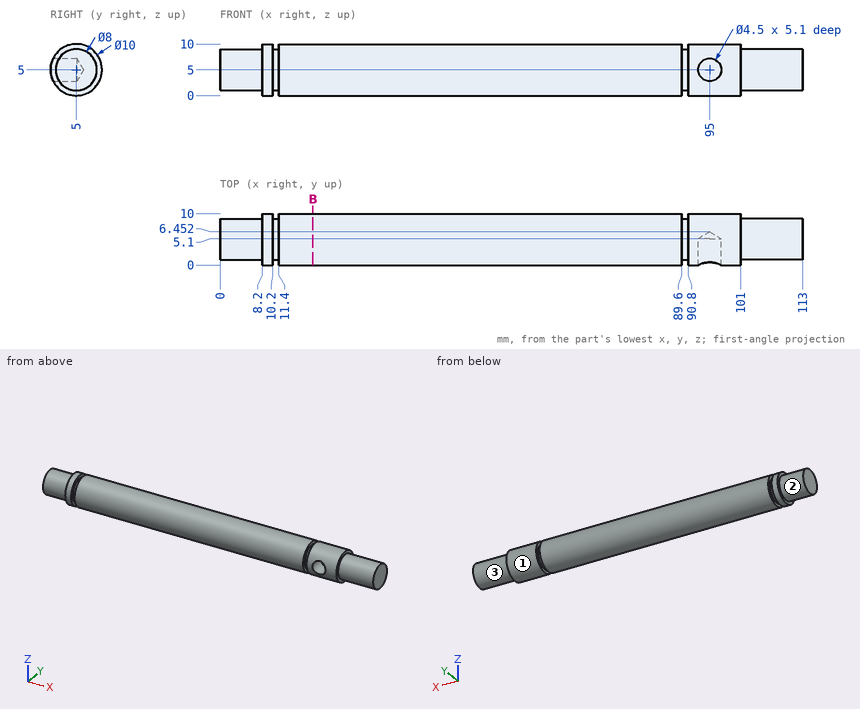
Can you work these out from the drawing? Everything is in mm from the part's minimum corner. A direction names the side the tool comes from. Round coordinates to 2 decimals unless told otherwise and drop trailing zeros. Loops run counter-clockwise (first coordinate to the right, second up) from the corner with the lowest first, then second, coordinate; pieces in that order, holes last. Notation, with made-up numbers: (-12, 38) -> (45, 38) arc R22 cw to (45, 70) -> close; hole circle Ø1 at (13.25, 45.25). An arc over 180 degrees is marked (long way). Answer in a Markdown table with one row per item.
Item 1: If I drill on probe 1 along X at (y, z) = (9, 4); probe 2 along X at (y, z) = (1.45, 5); probe 3 along X at (y, z) = (1.25, 6.5), over which ranges is the centre line in solid material (lowest first)?
Answer block:
| item | result |
|---|---|
| probe 1 | 8.2 to 10.2, 11.4 to 89.6, 90.8 to 101 |
| probe 2 | 0 to 92.75, 97.25 to 113 |
| probe 3 | 8.2 to 10.2, 11.4 to 89.6, 90.8 to 93.32, 96.68 to 101 |
Item 2: On a 3-axis mill with a long thin cutter (end or side, diameter ignored), from which of +Z, -Z, +X, -X, +Y, -Y can I reach the whole of each face in a straight line? I mean the marked faces 1, 2 and 3. Say none if no direction works.
Answer block:
| item | result |
|---|---|
| face 1 | +X, -X |
| face 2 | -X |
| face 3 | +X |
Item 3: Suppose I cut it at B-B, the plane x = 18. List the corners of the cut face in (y, z) for me, plus the area to 3 significant figures.
Answer block:
| item | result |
|---|---|
| outline | circle Ø10 at (5, 5) |
| area | 78.5 mm² |
Item 4: Will these pins go through, and if not, where does the flat tip stop? P1, Ø2, axis at x = 39, z = 5.5, coming from the -Y side; P2, Ø2, axis at x = 54.5, z = 2.5, coming from the -Y side; P3, Ø1, axis at x = 58.5, y = 1, coming from the -Z side; P4, Ø2, axis at x = 39, y = 7, coming from the +Z side.
Answer block:
| item | result |
|---|---|
| P1 | y = 0 |
| P2 | y = 0.23 |
| P3 | z = 1.43 |
| P4 | z = 9.9 |
